from build123d import *

# Parameters (mm, degrees)
F0_W     = 76.2
F0_H     = 38.1
F1_DEPTH = 6.35


with BuildPart() as f1:
    # F0 (on Top) → F1 (new body)
    with BuildSketch(Plane.XY):
        Rectangle(F0_W, F0_H)
        Polygon((-21.091462, 5.95622), (-17.652636, 7.941627), (-17.652636, 4.5851), (-14.29611, 4.5851), (-15.974373, 1.678263), (-13.067536, 0), (-16.506361, -1.985407), (-15.360086, -3.970813), (-17.652636, -3.970813), (-17.652636, -7.941627), (-20.559474, -6.263364), (-22.237737, -9.170201), (-23.916, -6.263364), (-26.822837, -7.941627), (-26.822837, -3.970813), (-29.115387, -3.970813), (-27.969112, -1.985407), (-31.407937, 0), (-28.5011, 1.678263), (-30.179363, 4.5851), (-26.822837, 4.5851), (-26.822837, 7.941627), (-23.384012, 5.95622), (-22.237737, 7.941627), align=None, mode=Mode.SUBTRACT)
    extrude(amount=F1_DEPTH)


solid = f1.part
Here's how the part is built. I have some questions about the finished solid (model axes, mm). A direction names the side the tool comes from. Coordinates: 2 decimals unless noted, no trailing zeros. Write each loop counter-clockwise with the first axis right and the second up, starting at its lowest first coordinate (ties: lowest second). Pieces come first, ordered by that corner, then holes. Notation, with made-up numbers: (22.5, 18) - (33.5, 18) arc R31 cw to (33.5, 46) - close; hole circle Ø11 at (51, 58). An arc over 180 degrees is marked (long way). Use one line per item in the form item = value.
1) Suppose I cut it at D-D, the plane y = -7. Write out the boundary of the cut face in (x, z), plus the area to 3 significant figures.
Solved:
outline = (-38.1, 0) - (-26.82, 0) - (-26.82, 6.35) - (-38.1, 6.35) - close; (-25.19, 0) - (-23.49, 0) - (-23.49, 6.35) - (-25.19, 6.35) - close; (-20.98, 0) - (-19.28, 0) - (-19.28, 6.35) - (-20.98, 6.35) - close; (-17.65, 0) - (38.1, 0) - (38.1, 6.35) - (-17.65, 6.35) - close
area = 447 mm2
2) Suppose I cut it at B-B, the plane x = -25.5. Write out the boundary of the cut face in (y, z), plus the area to 3 significant figures.
Solved:
outline = (-19.05, 0) - (-7.18, 0) - (-7.18, 6.35) - (-19.05, 6.35) - close; (7.18, 0) - (19.05, 0) - (19.05, 6.35) - (7.18, 6.35) - close
area = 151 mm2
3) On a 3-axis mill with a long thin cutter (end or side, diameter ignored), from which of +Z, -Z, +X, -X, +Y, -Y can I reach the whole of each face in a straight line? I mean faces 1 (the flat face through (-19.396, 6.935, 3.131)), 2 (the flat face through (-1, 0, 6.35)). Say none if no direction works.
Solved:
face_1 = +Z, -Z
face_2 = +Z, +X, -X, +Y, -Y
4) Thinking about a two-plate mould opening in Y: for faces 3 (the flat face through (-19.09, -7.11, 3.13)), 4 (the flat face through (-38.1, 0, 3)), 5 (the flat face through (-1, -19.05, 3)), 6 (the flat face through (-22.819, 6.935, 3.131)), which applies, released by +Y, released by -Y, zero draft, split by the parting line, or undercut?
Solved:
face_3 = undercut
face_4 = zero draft
face_5 = released by -Y
face_6 = undercut
5) Suppose I cut it at A-A, the plane z = 1.75. Write out the boundary of the cut face in (x, y).
Solved:
outline = (-38.1, -19.05) - (38.1, -19.05) - (38.1, 19.05) - (-38.1, 19.05) - close; hole (-31.41, 0) - (-27.97, -1.99) - (-29.12, -3.97) - (-26.82, -3.97) - (-26.82, -7.94) - (-23.92, -6.26) - (-22.24, -9.17) - (-20.56, -6.26) - (-17.65, -7.94) - (-17.65, -3.97) - (-15.36, -3.97) - (-16.51, -1.99) - (-13.07, 0) - (-15.97, 1.68) - (-14.3, 4.59) - (-17.65, 4.59) - (-17.65, 7.94) - (-21.09, 5.96) - (-22.24, 7.94) - (-23.38, 5.96) - (-26.82, 7.94) - (-26.82, 4.59) - (-30.18, 4.59) - (-28.5, 1.68) - close
6) I'm going to push a flat-ended pin straight in: P1, Ø6, axis at x = 10, y = -4.5, coming from the -Z side. Where does the tip first touch, or does it pass through?
Solved:
P1 = 0
7) I need wall thicknesses on line 1 (X direction, y = -6, z = 1.5); line 2 (Y direction, x = -15.5, z = 2); line 3 (X direction, y = -9, z = 1.75). Which ranges of each line are inside material? Lowest first, please.
Solved:
line_1 = -38.1 to -26.82, -17.65 to 38.1
line_2 = -19.05 to -3.97, -3.73 to -1.4, 1.4 to 2.5, 4.59 to 19.05
line_3 = -38.1 to -22.34, -22.14 to 38.1
8) Suppose I cut it at C-C, the plane y = 2.5. Write out the boundary of the cut face in (x, z), plus the area to 3 significant figures.
Solved:
outline = (-38.1, 0) - (-28.98, 0) - (-28.98, 6.35) - (-38.1, 6.35) - close; (-15.5, 0) - (38.1, 0) - (38.1, 6.35) - (-15.5, 6.35) - close
area = 398 mm2
